```python
from build123d import *

# Parameters (mm, degrees)
SKETCH1_W                 = 498.348
SKETCH1_H                 = 177.8
BOSS_EXTRUDE1_DEPTH       = 1.5875
BOSS_EXTRUDE2_DEPTH       = 3.175
SKETCH3_R                 = 5
CUT_EXTRUDE1_DEPTH        = 318.565245896
LPATTERN3_COUNT           = 3
LPATTERN3_PITCH           = 12.7
LPATTERN3_COL_COUNT       = 3
LPATTERN3_COL_PITCH       = 12.7
LPATTERN1_COUNT           = 2
LPATTERN1_PITCH           = 197.7136
LPATTERN1_COPY_1_SKETCH_R = 5
LPATTERN1_COPY_1_DEPTH    = 318.565245896
LPATTERN1_COPY_2_SKETCH_R = 5
LPATTERN1_COPY_2_DEPTH    = 318.565245896
LPATTERN1_COPY_3_SKETCH_R = 5
LPATTERN1_COPY_3_DEPTH    = 318.565245896
LPATTERN1_COPY_4_SKETCH_R = 5
LPATTERN1_COPY_4_DEPTH    = 318.565245896
SKETCH4_R                 = 5
CUT_EXTRUDE2_DEPTH        = 318.565245896
LPATTERN4_COUNT           = 3
LPATTERN4_PITCH           = 12.7
LPATTERN4_COL_COUNT       = 3
LPATTERN4_COL_PITCH       = 12.7
LPATTERN5_COUNT           = 4
LPATTERN5_PITCH           = 98.8568
LPATTERN5_COPY_1_SKETCH_R = 5
LPATTERN5_COPY_1_DEPTH    = 318.565245896
LPATTERN5_COPY_2_SKETCH_R = 5
LPATTERN5_COPY_2_DEPTH    = 318.565245896
LPATTERN5_COPY_3_SKETCH_R = 5
LPATTERN5_COPY_3_DEPTH    = 318.565245896
LPATTERN5_COPY_4_SKETCH_R = 5
LPATTERN5_COPY_4_DEPTH    = 318.565245896
LPATTERN5_COPY_5_SKETCH_R = 5
LPATTERN5_COPY_5_DEPTH    = 318.565245896
LPATTERN5_COPY_6_SKETCH_R = 5
LPATTERN5_COPY_6_DEPTH    = 318.565245896
LPATTERN5_COPY_7_SKETCH_R = 5
LPATTERN5_COPY_7_DEPTH    = 318.565245896
LPATTERN5_COPY_8_SKETCH_R = 5
LPATTERN5_COPY_8_DEPTH    = 318.565245896


with BuildPart() as part:
    # Sketch1 → Boss-Extrude1 (new, symmetric)
    with BuildSketch(Plane(origin=(0, 0, 0), x_dir=(0, 0, -1), z_dir=(1, 0, 0))):
        Rectangle(SKETCH1_W, SKETCH1_H)
    extrude(amount=BOSS_EXTRUDE1_DEPTH, both=True)

    # Sketch2 → Boss-Extrude2 (add)
    with BuildSketch(Plane(origin=(1.5875, 0, 0), x_dir=(0, 0, -1), z_dir=(1, 0, 0))):
        Polygon((249.174, -88.9), (48.2854, -88.9), (48.2854, -196.85), (149.8854, -196.85), (185.674, -101.6), (249.174, -101.6), align=None)
    extrude(amount=-BOSS_EXTRUDE2_DEPTH)

    # Sketch3 → Cut-Extrude1 (cut, through all)
    with BuildSketch(Plane(origin=(1.5875, 0, 0), x_dir=(0, 0, -1), z_dir=(1, 0, 0))):
        with Locations((155.3337, 27.7749)):
            Circle(SKETCH3_R)
    cut_extrude1 = extrude(amount=-CUT_EXTRUDE1_DEPTH, mode=Mode.SUBTRACT)

    # LPattern3: Cut-Extrude1 ×3
    with Locations(*[(0, i * LPATTERN3_PITCH, 0) for i in range(1, LPATTERN3_COUNT)]):
        add(cut_extrude1, mode=Mode.SUBTRACT)

    # LPattern3 col: Cut-Extrude1 ×3
    with Locations(*[(0, -i * LPATTERN3_COL_PITCH, 0) for i in range(1, LPATTERN3_COL_COUNT)]):
        add(cut_extrude1, mode=Mode.SUBTRACT)

    # LPattern1: Cut-Extrude1 ×2
    with Locations(*[(0, 0, i * LPATTERN1_PITCH) for i in range(1, LPATTERN1_COUNT)]):
        add(cut_extrude1, mode=Mode.SUBTRACT)

    # LPattern1 copy 1 sketch → LPattern1 copy 1 (cut, through all)
    with BuildSketch(Plane(origin=(1.5875, 12.7, 197.7136), x_dir=(0, 0, -1), z_dir=(1, 0, 0))):
        with Locations((155.3337, 27.7749)):
            Circle(LPATTERN1_COPY_1_SKETCH_R)
    extrude(amount=-LPATTERN1_COPY_1_DEPTH, mode=Mode.SUBTRACT)

    # LPattern1 copy 2 sketch → LPattern1 copy 2 (cut, through all)
    with BuildSketch(Plane(origin=(1.5875, 25.4, 197.7136), x_dir=(0, 0, -1), z_dir=(1, 0, 0))):
        with Locations((155.3337, 27.7749)):
            Circle(LPATTERN1_COPY_2_SKETCH_R)
    extrude(amount=-LPATTERN1_COPY_2_DEPTH, mode=Mode.SUBTRACT)

    # LPattern1 copy 3 sketch → LPattern1 copy 3 (cut, through all)
    with BuildSketch(Plane(origin=(1.5875, -12.7, 197.7136), x_dir=(0, 0, -1), z_dir=(1, 0, 0))):
        with Locations((155.3337, 27.7749)):
            Circle(LPATTERN1_COPY_3_SKETCH_R)
    extrude(amount=-LPATTERN1_COPY_3_DEPTH, mode=Mode.SUBTRACT)

    # LPattern1 copy 4 sketch → LPattern1 copy 4 (cut, through all)
    with BuildSketch(Plane(origin=(1.5875, -25.4, 197.7136), x_dir=(0, 0, -1), z_dir=(1, 0, 0))):
        with Locations((155.3337, 27.7749)):
            Circle(LPATTERN1_COPY_4_SKETCH_R)
    extrude(amount=-LPATTERN1_COPY_4_DEPTH, mode=Mode.SUBTRACT)

    # Sketch4 → Cut-Extrude2 (cut, through all)
    with BuildSketch(Plane(origin=(1.5875, 0, 0), x_dir=(0, 0, -1), z_dir=(1, 0, 0))):
        with Locations((141.2367, 27.7749)):
            Circle(SKETCH4_R)
    cut_extrude2 = extrude(amount=-CUT_EXTRUDE2_DEPTH, mode=Mode.SUBTRACT)

    # LPattern4: Cut-Extrude2 ×3
    with Locations(*[(0, i * LPATTERN4_PITCH, 0) for i in range(1, LPATTERN4_COUNT)]):
        add(cut_extrude2, mode=Mode.SUBTRACT)

    # LPattern4 col: Cut-Extrude2 ×3
    with Locations(*[(0, -i * LPATTERN4_COL_PITCH, 0) for i in range(1, LPATTERN4_COL_COUNT)]):
        add(cut_extrude2, mode=Mode.SUBTRACT)

    # LPattern5: Cut-Extrude2 ×4, 1 skipped
    with Locations(*[(0, 0, i * LPATTERN5_PITCH) for i in range(1, LPATTERN5_COUNT) if i not in (1,)]):
        add(cut_extrude2, mode=Mode.SUBTRACT)

    # LPattern5 copy 1 sketch → LPattern5 copy 1 (cut, through all)
    with BuildSketch(Plane(origin=(1.5875, 12.7, 197.7136), x_dir=(0, 0, -1), z_dir=(1, 0, 0))):
        with Locations((141.2367, 27.7749)):
            Circle(LPATTERN5_COPY_1_SKETCH_R)
    extrude(amount=-LPATTERN5_COPY_1_DEPTH, mode=Mode.SUBTRACT)

    # LPattern5 copy 2 sketch → LPattern5 copy 2 (cut, through all)
    with BuildSketch(Plane(origin=(1.5875, 12.7, 296.5704), x_dir=(0, 0, -1), z_dir=(1, 0, 0))):
        with Locations((141.2367, 27.7749)):
            Circle(LPATTERN5_COPY_2_SKETCH_R)
    extrude(amount=-LPATTERN5_COPY_2_DEPTH, mode=Mode.SUBTRACT)

    # LPattern5 copy 3 sketch → LPattern5 copy 3 (cut, through all)
    with BuildSketch(Plane(origin=(1.5875, 25.4, 197.7136), x_dir=(0, 0, -1), z_dir=(1, 0, 0))):
        with Locations((141.2367, 27.7749)):
            Circle(LPATTERN5_COPY_3_SKETCH_R)
    extrude(amount=-LPATTERN5_COPY_3_DEPTH, mode=Mode.SUBTRACT)

    # LPattern5 copy 4 sketch → LPattern5 copy 4 (cut, through all)
    with BuildSketch(Plane(origin=(1.5875, 25.4, 296.5704), x_dir=(0, 0, -1), z_dir=(1, 0, 0))):
        with Locations((141.2367, 27.7749)):
            Circle(LPATTERN5_COPY_4_SKETCH_R)
    extrude(amount=-LPATTERN5_COPY_4_DEPTH, mode=Mode.SUBTRACT)

    # LPattern5 copy 5 sketch → LPattern5 copy 5 (cut, through all)
    with BuildSketch(Plane(origin=(1.5875, -12.7, 197.7136), x_dir=(0, 0, -1), z_dir=(1, 0, 0))):
        with Locations((141.2367, 27.7749)):
            Circle(LPATTERN5_COPY_5_SKETCH_R)
    extrude(amount=-LPATTERN5_COPY_5_DEPTH, mode=Mode.SUBTRACT)

    # LPattern5 copy 6 sketch → LPattern5 copy 6 (cut, through all)
    with BuildSketch(Plane(origin=(1.5875, -12.7, 296.5704), x_dir=(0, 0, -1), z_dir=(1, 0, 0))):
        with Locations((141.2367, 27.7749)):
            Circle(LPATTERN5_COPY_6_SKETCH_R)
    extrude(amount=-LPATTERN5_COPY_6_DEPTH, mode=Mode.SUBTRACT)

    # LPattern5 copy 7 sketch → LPattern5 copy 7 (cut, through all)
    with BuildSketch(Plane(origin=(1.5875, -25.4, 197.7136), x_dir=(0, 0, -1), z_dir=(1, 0, 0))):
        with Locations((141.2367, 27.7749)):
            Circle(LPATTERN5_COPY_7_SKETCH_R)
    extrude(amount=-LPATTERN5_COPY_7_DEPTH, mode=Mode.SUBTRACT)

    # LPattern5 copy 8 sketch → LPattern5 copy 8 (cut, through all)
    with BuildSketch(Plane(origin=(1.5875, -25.4, 296.5704), x_dir=(0, 0, -1), z_dir=(1, 0, 0))):
        with Locations((141.2367, 27.7749)):
            Circle(LPATTERN5_COPY_8_SKETCH_R)
    extrude(amount=-LPATTERN5_COPY_8_DEPTH, mode=Mode.SUBTRACT)


solid = part.part
```
Input: part model. Units: mm. Frame: model coordinates. Give positions to 0.01 mm unless a question says otherwise; leave off trailing zeros. Order: outer loops, then holes, each group sorted by start corner. A loop starts at its lowest first (then second) coordinate and runs counter-clockwise, first axis right, second up. Notation, with made-up numbers: (-11.75, 59) - (22.25, 59) arc R31 cw to (22.25, 84) - close; hole circle Ø8 at (51.25, 21.25). An arc over 180 degrees is marked (long way). Use a Markdown table: item, result.
(1) Draft query along Z for faces 1 (the flat face through (1.588, -20, 3)), 2 (the cylindrical face through (0.02, 27.99, -150.34)), 3 (the cylindrical face through (0, 10.2, 43.5)). Return one class per face: released by +Z, released by -Z, zero draft, split by the parting line, or undercut.
Computed values:
| item | result |
|---|---|
| face 1 | zero draft |
| face 2 | undercut |
| face 3 | undercut |
(2) Section query B-B (z = 106). Output: boundary loops of the cut face in (x, y), then the cut area to 3 significant figures.
Computed values:
| item | result |
|---|---|
| outline | (-1.59, -88.9) - (1.59, -88.9) - (1.59, 88.9) - (-1.59, 88.9) - close |
| area | 565 mm2 |
(3) Section query A-A (x = 0.8). State how many separate pieces and enclosed holes the cut face has, then the cut area to 3 significant figures.
Computed values:
| item | result |
|---|---|
| separate pieces | 1 |
| enclosed holes | 25 |
| area | 101,000 mm2 |
(4) Line query: line 1 (Z direction, x = 1.4, y = 2); line 2 (Y direction, x = 0.3, z = -39); line 3 (Z direction, x = -0.55, y = 3.5). Output: solid intervals per line, ascending. Write a range as from..to.
Computed values:
| item | result |
|---|---|
| line 1 | z = -249.17..-160.32, -150.35..-146.22, -136.25..37.39, 47.37..51.49, 61.46..150.35, 160.32..249.17 |
| line 2 | y = -88.9..88.9 |
| line 3 | z = -249.17..-160.21, -150.46..-146.11, -136.36..37.51, 47.25..51.61, 61.35..150.46, 160.21..249.17 |
(5) Section query C-C (y = -147). Output: boundary loops of the cut face in (x, z), then the cut area to 3 significant figures.
Computed values:
| item | result |
|---|---|
| outline | (-1.59, -168.62) - (1.59, -168.62) - (1.59, -48.29) - (-1.59, -48.29) - close |
| area | 382 mm2 |
